Job drawing, mm, ordinate dimensions from the low corner. One solid piece. Coordinates: 2 decimals unless noted, no trailing zeros. Order: outer loops, then holes, each group sorted by start corner. A loop starts at its lowest first (then second) coordinate and runs counter-clockwise, first axis right, second up. Notation, with made-up numbers: (61.5, 25) - (97.5, 25) arc R33 ccw to (97.5, 64) - close; hole circle Ø11 at (71.25, 65). An arc over 180 degrees is marked (long way). Use a Markdown table: item, result. Add a question column.
1) Drop a flat-ended pin along its axis: P1, Ø1.9, axis at x = 196.825, y = 67.5, coming from the -Z side. Give the stop position or say it passes through.
2) Wall check: L1, parallel to Y at x = 35, z = 3.5 (3 decimals); L2, parallel to X at y = 19.5, z = 5.75; L3, parallel to Y at x = 84.5, z = 3.25. Give the ranges that are in metal, low to high. Write a range as [from, to].
3) Saw through at C-C on z = 1. Count the separate pieces of the cut face and the enclosed holes in it, then the cut area to 3 significant figures.
4) Saw through at A-A on x = 103. List the corners of the cut face in (y, z).
5) Saw through at B-B on y = 170. List the corners of the cut face in (x, z), then the cut area to 3 significant figures.
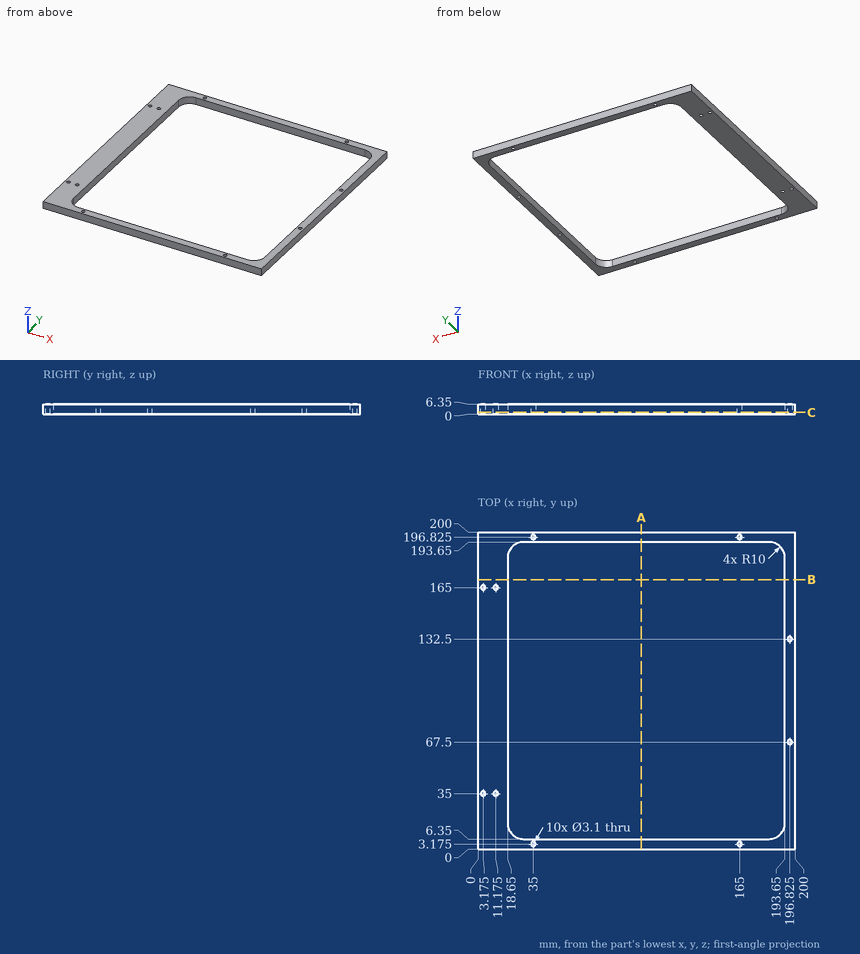
Results are:
| question | item | result |
|---|---|---|
| 1 | P1 | through |
| 2 | L1 | [0, 1.625], [4.725, 6.35], [193.65, 195.275], [198.375, 200] |
| 2 | L2 | [0, 18.65], [193.65, 200] |
| 2 | L3 | [0, 6.35], [193.65, 200] |
| 3 | separate pieces | 1 |
| 3 | enclosed holes | 11 |
| 3 | area | 7,230 mm2 |
| 4 | outline | (0, 0) - (6.35, 0) - (6.35, 6.35) - (0, 6.35) - close; (193.65, 0) - (200, 0) - (200, 6.35) - (193.65, 6.35) - close |
| 5 | outline | (0, 0) - (18.65, 0) - (18.65, 6.35) - (0, 6.35) - close; (193.65, 0) - (200, 0) - (200, 6.35) - (193.65, 6.35) - close |
| 5 | area | 159 mm2 |
